Can you work these out from the model? Positions are in its coordinate system, mm. A direction names the side the tool comes from. Coordinates: 2 decimals unless noted, no trailing zeros. Write each loop counter-clockwise with the first axis right and the second up, starting at its lowest first coordinate (ties: lowest second). Pieces come first, ordered by that corner, then holes. Notation, with made-up numbers: M 5.5,68 L 23.5,68 A29 cw 23.5,92 Z; hole C -37.5,-20 d6. An arc over 180 degrees is marked long. Use one line per item in the form item = value. Start each with the question number.
Solid Edge part; units mm, degrees
sketch "Sketch1" plane through (0, 0, 0) normal (0, 0, 1) x (1, 0, 0)
  circle A0 centre (0, 0) radius 3.5
extrude "Protrusion1" add sketch "Sketch1" along normal blind 4
sketch "Sketch2" plane through (0, 0, 0) normal (0, 0, -1) x (1, 0, 0)
  circle A0 centre (0, 0) radius 2
extrude "Protrusion2" add sketch "Sketch2" along normal blind 50
sketch "Sketch3" plane through (0, 0, -50) normal (0, 0, -1) x (1, 0, 0)
  circle A0 centre (0, 0) radius 1.9997
extrude "Cutout1" cut sketch "Sketch3" against normal blind 20 flip side to cut
chamfer "Chamfer_1" distance 0.3 angle 45 1 edges at (-1.9997, 0, -50)
sketch "Sketch4" plane through (0, 0, 4) normal (0, 0, 1) x (1, 0, 0)
  line L0 (-0.866, 1.5) -> (0.866, 1.5)
  line L1 (1.7321, 0) -> (0.866, 1.5)
  line L2 (0.866, -1.5) -> (1.7321, 0)
  line L3 (-0.866, -1.5) -> (0.866, -1.5)
  line L4 (-1.7321, 0) -> (-0.866, -1.5)
  line L5 (-0.866, 1.5) -> (-1.7321, 0)
extrude "Cutout2" cut sketch "Sketch4" against normal blind 2
properties part number "24101455"
1) Suppose I cut it at B-B on z = -41. Please give me the cut outline in (x, y), and give its area (3 significant figures).
2) Suppose I cut it at C-C on y = -2.5. Please give me the cut outline in (x, z).
3) If we mould it in two halves opening along X, with no side actions, what happens to faces 4 (the face through (3.233, 1.341, 1.972)), 5 (the face through (-1.305, -0.74, 3.014)), 6 (the face through (0, -2, 4))? For each: +X half, -X half, draft (parallel to the pull), parting line (faces both ways), or undercut.
4) Will these pins go through, and if not, where does the flat tip stop? pin 1 Ø0.5 at (x, z) = (0.5, 3) entering from +Y; pin 2 Ø4 at (x, z) = (-2, -36) entering from -Y; pin 3 Ø4 at (x, z) = (0, -5.5) entering from +Y.
5) Please list where these lines run through material, in increasing order: line 1 (Z direction, x = 1, y = 1); line 2 (Z direction, x = -2.75, y = 1.5); line 3 (Y direction, x = -2, z = 1.5).
6) Which directions (+Z, -Z, +X, -X, +Y, -Y) give clear straight access to the entire face, cutting with the end or side of a thin tool? Please do faces 1 (the face through (0, 0, -50)), 2 (the face through (2, -2, 0)), 3 (the face through (1.293, -0.76, 3.014)).
Computed values:
q1.outline = C 0,0 d4
q1.area = 12.6 mm²
q2.outline = M -2.45,0 L 2.45,0 L 2.45,4 L -2.45,4 Z
q3.face_4 = parting line
q3.face_5 = undercut
q3.face_6 = draft
q4.pin_1 = 3.49
q4.pin_2 = -2
q4.pin_3 = 2
q5.line_1 = -50 to 2
q5.line_2 = 0 to 4
q5.line_3 = -2.87 to 2.87
q6.face_1 = -Z, +X, -X, +Y, -Y
q6.face_2 = -Z
q6.face_3 = +Z
